from build123d import *

# Parameters (mm, degrees)
SKETCH1_W           = 150.5
SKETCH1_H           = 90.5
BOSS_EXTRUDE1_DEPTH = 3
SKETCH2_W           = 150.5
SKETCH2_H           = 90.5
SKETCH2_W_2         = 137.5
SKETCH2_H_2         = 84.5
BOSS_EXTRUDE2_DEPTH = 11
SKETCH3_R           = 1.5
CUT_EXTRUDE1_DEPTH  = 31
SKETCH4_R           = 3
CUT_EXTRUDE2_DEPTH  = 3.5
SKETCH5_W           = 32
SKETCH5_H           = 14
SKETCH5_W_2         = 42
SKETCH5_W_3         = 44
SKETCH5_H_2         = 6
SKETCH5_W_4         = 45
SKETCH5_W_5         = 20
SKETCH5_H_3         = 20
SKETCH5_W_6         = 14
SKETCH5_H_4         = 5
SKETCH5_W_7         = 10
SKETCH5_H_5         = 10
CUT_EXTRUDE3_DEPTH  = 15
SKETCH7_W           = 40
SKETCH7_H           = 9
CUT_EXTRUDE4_DEPTH  = 15


with BuildPart() as part:
    # Sketch1 → Boss-Extrude1 (new body)
    with BuildSketch(Plane(origin=(0, 0, 0), x_dir=(1, 0, 0), z_dir=(0, 1, 0))):
        Rectangle(SKETCH1_W, SKETCH1_H)
    extrude(amount=BOSS_EXTRUDE1_DEPTH)

    # Sketch2 → Boss-Extrude2 (add)
    with BuildSketch(Plane(origin=(0, 0, 0), x_dir=(-1, 0, 0), z_dir=(0, -1, 0))):
        Rectangle(SKETCH2_W, SKETCH2_H)
        Rectangle(SKETCH2_W_2, SKETCH2_H_2, mode=Mode.SUBTRACT)
    extrude(amount=BOSS_EXTRUDE2_DEPTH)

    # Sketch3 → Cut-Extrude1 (cut)
    with BuildSketch(Plane(origin=(0, 3, 0), x_dir=(1, 0, 0), z_dir=(0, 1, 0))):
        with Locations(Location((-71.5, 41.25, 0), (0, 0, 270))):
            Circle(SKETCH3_R)
        with Locations(Location((-71.5, -41.25, 0), (0, 0, 270))):
            Circle(SKETCH3_R)
        with Locations(Location((71.5, -41.25, 0), (0, 0, 270))):
            Circle(SKETCH3_R)
        with Locations(Location((71.5, 41.25, 0), (0, 0, 270))):
            Circle(SKETCH3_R)
    extrude(amount=-CUT_EXTRUDE1_DEPTH, mode=Mode.SUBTRACT)

    # Sketch4 → Cut-Extrude2 (cut)
    with BuildSketch(Plane(origin=(0, 3, 0), x_dir=(1, 0, 0), z_dir=(0, 1, 0))):
        with Locations(Location((-71.5, 41.25, 0), (0, 0, 270))):
            Circle(SKETCH4_R)
        with Locations(Location((-71.5, -41.25, 0), (0, 0, 270))):
            Circle(SKETCH4_R)
        with Locations(Location((71.5, -41.25, 0), (0, 0, 270))):
            Circle(SKETCH4_R)
        with Locations(Location((71.5, 41.25, 0), (0, 0, 270))):
            Circle(SKETCH4_R)
    extrude(amount=-CUT_EXTRUDE2_DEPTH, mode=Mode.SUBTRACT)

    # Sketch5 → Cut-Extrude3 (cut)
    with BuildSketch(Plane(origin=(0, 3, 0), x_dir=(1, 0, 0), z_dir=(0, 1, 0))):
        with Locations((-51.25, -38.25)):
            Rectangle(SKETCH5_W, SKETCH5_H)
        with Locations((-2.25, -38.25)):
            Rectangle(SKETCH5_W_2, SKETCH5_H)
        with Locations((42.75, -37.25)):
            Rectangle(SKETCH5_W_3, SKETCH5_H_2)
        with Locations((42.75, 38.25)):
            Rectangle(SKETCH5_W_4, SKETCH5_H)
        with Locations((3.25, 18.25)):
            Rectangle(SKETCH5_W_5, SKETCH5_H_3)
        with Locations((-58.25, 36.75)):
            Rectangle(SKETCH5_W_6, SKETCH5_H_4)
        with Locations((-53.744307693, 1.912180937)):
            Rectangle(SKETCH5_W_7, SKETCH5_H_5)
    extrude(amount=-CUT_EXTRUDE3_DEPTH, mode=Mode.SUBTRACT)

    # Sketch7 → Cut-Extrude4 (cut)
    with BuildSketch(Plane.ZY.offset(75.25)):
        with Locations((-14.171893674, -6.5)):
            Rectangle(SKETCH7_W, SKETCH7_H)
    extrude(amount=-CUT_EXTRUDE4_DEPTH, mode=Mode.SUBTRACT)


solid = part.part
Check sheet for the modelled part. Datum: model origin and axes. Units: mm. A direction names the side the tool comes from. Round coordinates to 2 decimals unless told otherwise and drop trailing zeros. Loops run counter-clockwise (first coordinate to the right, second up) from the corner with the lowest first, then second, coordinate; pieces in that order, holes last. Notation, with made-up numbers: M 44.25,84.5 L 73.25,84.5 A12 ccw 73.25,98.5 Z; hole C 55.5,73.25 d2. An arc over 180 degrees is marked long. One line per item, written item: value.
(1) Access from +Z, -Z, +X, -X, +Y, -Y to the whole of each face (thin tool, end or side, straight path). Record for faces 4 (the face through (-68.75, -4, 10)), 5 (the face through (20.75, 2, 37)), 6 (the face through (42, 2, -31.25)), 7 (the face through (-35.25, -1, 43)), 8 (the face through (-72, -2, -14)).
Computed values:
face 4: -Y
face 5: +Y, -Y
face 6: -Z, +Y, -Y
face 7: +Z, +Y, -Y
face 8: -X, -Y
(2) Sectioned sample at C-C, the plane x = 71.5. Record the cut outline in (y, z), then the cut area to 3 significant figures.
Computed values:
outline: M -11,-45.25 L 3,-45.25 L 3,-44.25 L -0.5,-44.25 L -0.5,-42.75 L -11,-42.75 Z; M -11,-39.75 L -0.5,-39.75 L -0.5,-38.25 L 3,-38.25 L 3,38.25 L -0.5,38.25 L -0.5,39.75 L -11,39.75 Z; M -11,42.75 L -0.5,42.75 L -0.5,44.25 L 3,44.25 L 3,45.25 L -11,45.25 Z
area: 1,160 mm^2
(3) Release check for a two-part mould opening along Z. For faces 1 (the face through (74.474, 1.274, -41.641)), 2 (the face through (-71, -4, 45.25)), 3 (the face through (20.25, -1, -43)) record: +Z half, -Z half, draft (parallel to the pull), parting line (faces both ways), or undercut.
Computed values:
face 1: undercut
face 2: +Z half
face 3: draft
(4) Sectioned sample at B-B, the plane z = -1. Record the cut outline in (x, y).
Computed values:
outline: M -75.25,-2 L -68.75,-2 L -68.75,0 L -58.74,0 L -58.74,3 L -75.25,3 Z; M -48.74,0 L 68.75,0 L 68.75,-11 L 75.25,-11 L 75.25,3 L -48.74,3 Z
(5) Sectioned sample at D-D, the plane z = 22. Record the cut outline in (x, y), then the cut area to 4 significant figures.
Computed values:
outline: M -75.25,-11 L -68.75,-11 L -68.75,0 L 68.75,0 L 68.75,-11 L 75.25,-11 L 75.25,3 L -75.25,3 Z
area: 594.5 mm^2
(6) Thickness scan on line 1 (Z direction, x = -71.5, y = -6.75); line 2 (Z direction, x = 71.5, y = -6.75); line 3 (Z direction, x = -71.5, y = 1.85). Record the ranges inside material, lowest first.
Computed values:
line 1: z = -45.25 to -42.75, -39.75 to -34.17, 5.83 to 39.75, 42.75 to 45.25
line 2: z = -45.25 to -42.75, -39.75 to 39.75, 42.75 to 45.25
line 3: z = -45.25 to -44.25, -38.25 to 38.25, 44.25 to 45.25
(7) Depth check by flat-ended pin: pin 1 Ø1.7 at (x, z) = (-70, 40.5) entering from +Y; pin 2 Ø2.5 at (x, z) = (-71.5, 41.25) entering from +Y; pin 3 Ø2 at (x, z) = (-72, -22) entering from -Y; pin 4 Ø12 at (x, z) = (-53.5, 31) entering from -Y. Enter the tip coordinate at first touch or a pass-through.
Computed values:
pin 1: stops at y = -0.5
pin 2: passes through
pin 3: stops at y = -2
pin 4: stops at y = 0
(8) Sectioned sample at A-A, the plane x = 0.5. Record the cut outline in (y, z).
Computed values:
outline: M -11,-45.25 L 3,-45.25 L 3,-28.25 L 0,-28.25 L 0,-42.25 L -11,-42.25 Z; M 0,-8.25 L 3,-8.25 L 3,31.25 L 0,31.25 Z
